Design review of the part built by this model. Coordinates are the model's own, in mm. Round coordinates to 2 decimals unless told otherwise and drop trailing zeros. Loops run counter-clockwise (first coordinate to the right, second up) from the corner with the lowest first, then second, coordinate; pieces in that order, holes last. Notation, with made-up numbers: (4, 49) - (58, 49) arc R24 ccw to (58, 78) - close; hole circle Ø2 at (26, 18). An arc over 180 degrees is marked (long way). Return JSON: item names as keys, results as strings. Group by question number.
(1) Wall thickness on L1, parallel to Y at x = 5.5, z = -2.75; L2, parallel to Z at x = 6.25, y = 3.25; L3, parallel to Z at x = 8, y = 3: over which ranges is each line inside the solid? List them lowest first. Write a range as [from, to].
(2) The part is to be moulded in two halves that separate along Y. For faces 1 (the cylindrical face through (4.93, -0.582, -4.127)), 2 (the flat face through (0, 2.1, 1.1)), say which applies: pulls with the +Y half, pulls with the -Y half, needs draft (parallel to the pull), parting line crosses it, or undercut.
(3) Clearance check with flat-ended pins moving along their axes: pin 1 (2 mm diameter, centred on x = 4.5, z = 0, fed in from +Y); pin 2 (1.5 mm diameter, centred on x = 1, y = -3, fed in from -Z); pin 3 (5 mm diameter, centred on x = 7.5, z = -3, fed in from +Y). State where each tip first meets the part, or that it passes through.
(4) We need section C-C, the plane z = 4. Write out the cut boundary in (x, y), and give its area (3 significant figures).
(5) We need section A-A, the plane y = 0. Write out the cut boundary in (x, z), and give its area (3 significant figures).
from build123d import *

# Parameters (mm, degrees)
BASPROSKE_W                                     = 10
BASPROSKE_H                                     = 4.9
TOOTHCUT_DEPTH                                  = 13.166347028
TEETHCUTS_COUNT                                 = 12
TEETHCUTS_ANGLE                                 = 330
BORSKE_R                                        = 0.5
BORE_DEPTH                                      = 50.0000508
SKETCH2_R                                       = 1
CUT_EXTRUDE1_DEPTH                              = 13.070224944
CSK_FOR_M2_FLAT_HEAD_MACHINE_SCREW1_D           = 2.4
CSK_FOR_M2_FLAT_HEAD_MACHINE_SCREW1_CSINK_D     = 4.4
CSK_FOR_M2_FLAT_HEAD_MACHINE_SCREW1_CSINK_ANGLE = 90


with BuildPart() as part:
    # BasProSke → Base-Revolve (revolve)
    with BuildSketch(Plane(origin=(0, 0, 0), x_dir=(1, 0, 0), z_dir=(0, 1, 0)), mode=Mode.PRIVATE) as base_revolve_sk:
        with Locations((5, 2.45)):
            Rectangle(BASPROSKE_W, BASPROSKE_H)
    revolve(base_revolve_sk.sketch.rotate(Axis((-10, 0, 0), (1, 0, 0)), 180), axis=Axis((-10, 0, 0), (1, 0, 0)))

    # TooCutSke → ToothCut (cut, through all)
    with BuildSketch(Plane(origin=(0, 0, 0), x_dir=(0, 0, -1), z_dir=(1, 0, 0))):
        with BuildLine():
            ThreePointArc((0.45535744, 3.292662388), (0, 3.324), (-0.45535744, 3.292662388))
            ThreePointArc((-0.45535744, 3.292662388), (-0.583649315, 4.130986789), (-1.105088241, 4.799827615))
            ThreePointArc((-1.105088241, 4.799827615), (0, 4.9254), (1.105088241, 4.799827615))
            ThreePointArc((1.105088241, 4.799827615), (0.583649315, 4.130986789), (0.45535744, 3.292662388))
        make_face()
    toothcut = extrude(amount=TOOTHCUT_DEPTH, mode=Mode.SUBTRACT)

    # TeethCuts: ToothCut ×12 about axis
    teethcuts_axis = Axis((-10, 0, 0), (1, 0, 0))
    for i in range(1, TEETHCUTS_COUNT):
        add(toothcut.rotate(teethcuts_axis, i * TEETHCUTS_ANGLE / (TEETHCUTS_COUNT - 1)), mode=Mode.SUBTRACT)

    # BorSke → Bore (cut, symmetric)
    with BuildSketch(Plane(origin=(0, 0, 0), x_dir=(0, 0, -1), z_dir=(1, 0, 0))):
        with Locations(Location((0, 0, 0), (0, 0, 180))):
            Circle(BORSKE_R)
    extrude(amount=BORE_DEPTH, both=True, mode=Mode.SUBTRACT)

    # Sketch2 → Cut-Extrude1 (cut, through all)
    with BuildSketch(Plane.ZY):
        Circle(SKETCH2_R)
    extrude(amount=-CUT_EXTRUDE1_DEPTH, mode=Mode.SUBTRACT)

    # CSK for M2 Flat Head Machine Screw1 (through all)
    with Locations(Plane.ZY):
        with Locations((0, 0)):
            CounterSinkHole(CSK_FOR_M2_FLAT_HEAD_MACHINE_SCREW1_D / 2, CSK_FOR_M2_FLAT_HEAD_MACHINE_SCREW1_CSINK_D / 2, counter_sink_angle=CSK_FOR_M2_FLAT_HEAD_MACHINE_SCREW1_CSINK_ANGLE)


solid = part.part
Solutions:
{
 "1": {"L1": "[-3.4, -2.1], [-1.87, 1.87], [2.1, 3.4]", "L2": "[-3.59, -2.52], [-1.36, 1.36], [2.52, 3.59]", "L3": "[-3.52, -2.27], [-1.43, 1.43], [2.27, 3.52]"},
 "2": {"face 1": "undercut", "face 2": "needs draft"},
 "3": {"pin 1": "y = 4.71", "pin 2": "z = -3.6", "pin 3": "y = 4.78"},
 "4": {"outline": "(0, -1.57) - (10, -1.57) - (10, -0.53) - (0, -0.53) - close; (0, 0.53) - (10, 0.53) - (10, 1.57) - (0, 1.57) - close", "area": "20.7 mm^2"},
 "5": {"outline": "(0, -3.32) - (10, -3.32) - (10, -1.2) - (1, -1.2) - (0, -2.2) - close; (0, 2.2) - (1, 1.2) - (10, 1.2) - (10, 3.32) - (0, 3.32) - close", "area": "41.5 mm^2"}
}
